from build123d import *

# Parameters (mm, degrees)
F2_R      = 2.5
F3_DEPTH  = 3
F4_W      = 3
F4_H      = 3
F4_W_2    = 41
F4_H_2    = 35
F5_DEPTH  = 114
F6_R      = 2.5
F7_DEPTH  = 3
F8_W      = 110
F8_H      = 20
F9_DEPTH  = 3
F10_W     = 47
F10_H     = 26
F10_W_2   = 48
F10_H_2   = 28
F11_DEPTH = 3
F13_DEPTH = 3
F14_SIZE  = 1


with BuildPart() as f3:
    # F2 (on Right) → F3 (new body)
    with BuildSketch(Plane.YZ):
        with BuildLine():
            ThreePointArc((22.5, 35), (21.0355339059, 38.5355339059), (17.5, 40))
            Line((17.5, 40), (-19.5, 40))
            ThreePointArc((-19.5, 40), (-23.0355339059, 38.5355339059), (-24.5, 35))
            Line((-24.5, 35), (-24.5, -38))
            Line((-24.5, -38), (22.5, -38))
            Line((22.5, -38), (22.5, 35))
        make_face()
        with Locations((-12, 34.5)):
            Circle(F2_R, mode=Mode.SUBTRACT)
        with Locations((10, 34.5)):
            Circle(F2_R, mode=Mode.SUBTRACT)
    extrude(amount=F3_DEPTH)

    # F4 (on Right) → F5 (join)
    with BuildSketch(Plane.YZ):
        with Locations((21, -36.5)):
            Rectangle(F4_W, F4_H)
        with Locations((-1, -36.5)):
            Rectangle(F4_W_2, F4_H)
        with Locations((21, -17.5)):
            Rectangle(F4_W, F4_H_2)
        with Locations((-23, -36.5)):
            Rectangle(F4_W, F4_H)
        with Locations((-23, -17.5)):
            Rectangle(F4_W, F4_H_2)
    extrude(amount=-F5_DEPTH)

    # F6 (on face) → F7 (join)
    with BuildSketch(Plane(origin=(-114, 0, 0), x_dir=(0, -1, 0), z_dir=(-1, 0, 0))):
        with BuildLine():
            ThreePointArc((24.5, 35), (23.0355339059, 38.5355339059), (19.5, 40))
            Line((19.5, 40), (-17.5, 40))
            ThreePointArc((-17.5, 40), (-21.0355339059, 38.5355339059), (-22.5, 35))
            Line((-22.5, 35), (-22.5, -38))
            Line((-22.5, -38), (24.5, -38))
            Line((24.5, -38), (24.5, 35))
        make_face()
        with Locations((-10, 34.5)):
            Circle(F6_R, mode=Mode.SUBTRACT)
    extrude(amount=F7_DEPTH)

    # F8 (on face) → F9 (join)
    with BuildSketch(Plane.XZ.offset(24.5)):
        with Locations((-57, 10)):
            Rectangle(F8_W, F8_H)
    extrude(amount=-F9_DEPTH)

    # F10 (on face) → F11 (cut, through all)
    with BuildSketch(Plane.XZ.offset(24.5)):
        with Locations((-85.5, -19)):
            Rectangle(F10_W, F10_H)
        with Locations((-28.5, -19)):
            Rectangle(F10_W_2, F10_H_2)
    extrude(amount=-F11_DEPTH, mode=Mode.SUBTRACT)

    # F12 (on face) → F13 (cut, through all)
    with BuildSketch(Plane(origin=(0, 22.5, 0), x_dir=(-1, 0, 0), z_dir=(0, 1, 0))):
        with BuildLine():
            ThreePointArc((85, -26), (85.5857864376, -27.4142135624), (87, -28))
            Line((87, -28), (95, -28))
            ThreePointArc((95, -28), (96.4142135624, -27.4142135624), (97, -26))
            Line((97, -26), (97, -24))
            ThreePointArc((97, -24), (96.4142135624, -22.5857864376), (95, -22))
            Line((95, -22), (87, -22))
            ThreePointArc((87, -22), (85.5857864376, -22.5857864376), (85, -24))
            Line((85, -24), (85, -26))
        make_face()
    extrude(amount=-F13_DEPTH, mode=Mode.SUBTRACT)

    # F14
    f14_edges = [f3.edges().sort_by_distance(p)[0] for p in [
        (-57, -24.5, -38),
        (3, -1, -38),
        (-57, 22.5, -38),
        (-117, -1, -38),
    ]]
    chamfer(f14_edges, length=F14_SIZE)


solid = f3.part
Check sheet for the modelled part. Datum: model origin and axes. Units: mm. A direction names the side the tool comes from. Round coordinates to 2 decimals unless told otherwise and drop trailing zeros. Loops run counter-clockwise (first coordinate to the right, second up) from the corner with the lowest first, then second, coordinate; pieces in that order, holes last.
1. Set-up check for faces 4 (the flat face through (-86, -23, -6)), 5 (the flat face through (-56, 19.5, -18)), 6 (the cylindrical face through (-115, 12, 36)), 7 (the flat face through (-56, 21, 0)), 8 (the flat face through (-58, -23, 20)): record each of +Z, -Z, +X, -X, +Y, -Y from which the full face is reachable in a straight line by a thin tool's end or side.
2. Sectioned sample at A-A on x = -8.5. Record the boundary of the cut face in (y, z), and give its area (3 significant figures).
3. Sectioned sample at D-D on z = 27.5. Record the boundary of the cut face in (x, y).
4. Sectioned sample at C-C on x = -91. Record the boundary of the cut face in (y, z), and give its area (3 significant figures).
5. Sectioned sample at B-B on y = -12. Record the boundary of the cut face in (x, z).
6. Mould release check, pull along Y, two halves, no side actions. Record for faces 1 (the flat face through (-56, -21.5, -2)), 2 (the flat face through (-56, -24.5, -10)), 3 (the flat face through (-2, -23, 10)): released by +Y, released by -Y, zero draft, split by the parting line, or undercut.
7. Gauge pin test, flat ends, axial feed: pin 1 Ø0.6 at (x, y) = (-1, -22.5) entering from +Z; pin 2 Ø1.5 at (x, y) = (-19.5, -22.5) entering from +Z; pin 3 Ø4 at (x, z) = (-93.5, 9.5) entering from +Y. Record the tip position at first contact, or that the pin passes through.
8. Scan lines: probe 1 along Z at (x, y) = (2, -12); probe 2 along X at (y, z) = (8.5, -7.5); probe 3 along Y at (x, z) = (1, 34). Record each from-to range of solid material in increasing order.
Recorded:
1. face 4: -Y
1. face 5: +Z
1. face 6: +X, -X
1. face 7: +Z, +Y
1. face 8: +Z, +Y, -Y
2. outline: (-24.5, -37) - (-23.5, -38) - (21.5, -38) - (22.5, -37) - (22.5, 0) - (19.5, 0) - (19.5, -35) - (-21.5, -35) - (-21.5, -33) - (-24.5, -33) - close; (-24.5, -5) - (-21.5, -5) - (-21.5, 20) - (-24.5, 20) - close
2. area: 326 mm2
3. outline: (-117, -24.5) - (-114, -24.5) - (-114, 22.5) - (-117, 22.5) - close; (0, -24.5) - (3, -24.5) - (3, 22.5) - (0, 22.5) - close
4. outline: (-24.5, -37) - (-23.5, -38) - (21.5, -38) - (22.5, -37) - (22.5, -28) - (19.5, -28) - (19.5, -35) - (-21.5, -35) - (-21.5, -32) - (-24.5, -32) - close; (-24.5, -6) - (-21.5, -6) - (-21.5, 20) - (-24.5, 20) - close; (19.5, -22) - (22.5, -22) - (22.5, 0) - (19.5, 0) - close
4. area: 314 mm2
5. outline: (-117, -37) - (-116, -38) - (2, -38) - (3, -37) - (3, 32) - (0, 32) - (0, -35) - (-114, -35) - (-114, 40) - (-117, 40) - close; (0, 37) - (3, 37) - (3, 40) - (0, 40) - close
6. face 1: undercut
6. face 2: released by -Y
6. face 3: zero draft
7. pin 1: stops at z = 0
7. pin 2: stops at z = 20
7. pin 3: stops at y = -21.5
8. probe 1: z = -38 to 32, 37 to 40
8. probe 2: x = -117 to -114, 0 to 3
8. probe 3: y = -24.5 to -14.45, -9.55 to 7.55, 12.45 to 22.5
